from build123d import *

# Parameters (mm, degrees)
ESTRUSIONE_ESTRUSIONE1_DEPTH   = 21
FORO_FILETTATO_M18X1_5_1_D     = 16.5
FORO_FILETTATO_M18X1_5_1_DEPTH = 38.542899893
FORO_FILETTATO_M18X1_5_1_TIP   = 4.957100107


with BuildPart() as part:
    # Schizzo1 → Estrusione-Estrusione1 (new, symmetric)
    with BuildSketch(Plane.XY):
        Polygon((30, 0), (30, 50), (15, 50), (-30, 30), (-30, 0), align=None)
    extrude(amount=ESTRUSIONE_ESTRUSIONE1_DEPTH, both=True)

    # Foro filettato M18x1.5-1
    with Locations(Plane(origin=(30, 0, 0), x_dir=(0, 0, -1), z_dir=(1, 0, 0))):
        with Locations((0, 25)):
            Hole(FORO_FILETTATO_M18X1_5_1_D / 2, depth=FORO_FILETTATO_M18X1_5_1_DEPTH)
            with Locations((0, 0, -(FORO_FILETTATO_M18X1_5_1_DEPTH + FORO_FILETTATO_M18X1_5_1_TIP / 2))):  # 118° drill point
                Cone(0, FORO_FILETTATO_M18X1_5_1_D / 2, FORO_FILETTATO_M18X1_5_1_TIP, mode=Mode.SUBTRACT)


solid = part.part
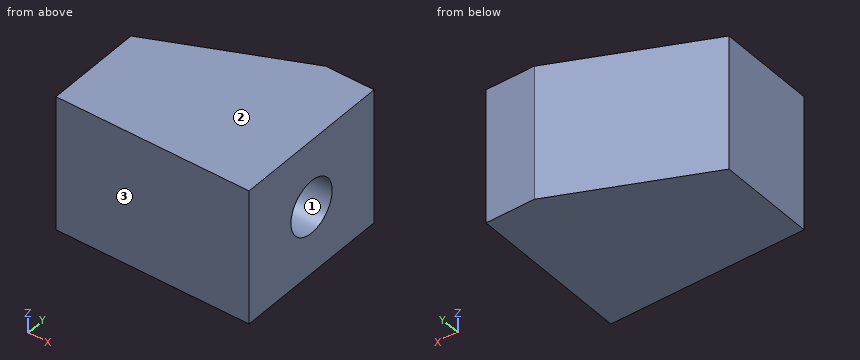
CAD build for the part. Positions are in the model's coordinates, mm. Face numbers are marked on the shaded views. Give positions to 0.01 mm unless a question says otherwise; leave off trailing zeros. Write each loop counter-clockwise with the first axis right and the second up, starting at its lowest first coordinate (ties: lowest second). Pieces come first, ordered by that corner, then holes. Notation, with made-up numbers: (72.5, 30) - (80.5, 30) arc R14 cw to (80.5, 36) - close; hole circle Ø5 at (50.25, -1). An arc over 180 degrees is marked (long way). Answer as CSV lines item,"result".
Q1. Band-saw the part on B-B (z = 10). Give the cut face in (x, y).
Result set:
outline,"(-30, 0) - (30, 0) - (30, 50) - (15, 50) - (-30, 30) - close"
Q2. Drill centre lines: line 1 (Z direction, x = 6, y = 25); line 2 (Y direction, x = 20, z = 0); line 3 (Y direction, x = -1.5, z = -3). Where is each one in solid material? Low to high. Write a range as from..to.
Result set:
line 1,"-21..-8.25, 8.25..21"
line 2,"0..16.75, 33.25..50"
line 3,"0..17.31, 32.69..42.67"
Q3. Band-saw the part on A-A (x = 25). Give the cut face in (y, z), and give its area (3 significant figures).
Result set:
outline,"(0, -21) - (50, -21) - (50, 21) - (0, 21) - close; hole circle Ø16.5 at (25, 0)"
area,"1,890 mm²"
Q4. Pull direction Y, two halves, no side cores. Call the marked faces 1, 2 and 3: released by +Y, released by -Y, zero draft, split by the parting line, or undercut.
Result set:
face 1,"undercut"
face 2,"zero draft"
face 3,"released by -Y"
Q5. Band-saw the part on D-D (x = 4.5). Give the cut face in (y, z), and give its area (3 significant figures).
Result set:
outline,"(0, -21) - (45.33, -21) - (45.33, 21) - (0, 21) - close; hole circle Ø16.5 at (25, 0)"
area,"1,690 mm²"
Q6. Flat gauge pins, fed straight in: pin 1 Ø2 at (y, z) = (36.5, -10.5) entering from -X (3 decimals); pin 2 Ø6 at (x, z) = (-4, -14.5) entering from +Y; pin 3 Ø4 at (y, z) = (43.5, -5) entering from -X (3 decimals); pin 4 Ø12 at (x, z) = (-4.5, -3.5) entering from -Y. Where does each tip first touch, or does it go through?
Result set:
pin 1,"x = -17.625"
pin 2,"y = 42.89"
pin 3,"x = -4.125"
pin 4,"y = 0"
Q7. Band-saw the part on C-C (y = 44). Give the cut face in (x, z).
Result set:
outline,"(1.5, -21) - (30, -21) - (30, 21) - (1.5, 21) - close"
